```python
from build123d import *

# Parameters (mm, degrees)
F1_DEPTH = 12
F3_W     = 10
F3_H     = 2
F4_DEPTH = 43
F6_W     = 9
F6_H     = 4.75
F7_DEPTH = 69
F9_D     = 3.5
F9_DEPTH = 4
F9_TIP   = 1.0515060833


with BuildPart() as f1:
    # F0 (on Front) → F1 (new body)
    with BuildSketch(Plane.XZ):
        Polygon((29.6939597434, -5.2816280767), (-18.3060402566, -5.2816280767), (-18.3060402566, -14.0816280767), (29.6939597434, -14.0816280767), (29.6939597434, -10.5816280767), (27.6939597434, -10.5816280767), (27.6939597434, -11.5816280767), (-16.3060402566, -11.5816280767), (-16.3060402566, -8.2816280767), (27.6939597434, -8.2816280767), (27.6939597434, -9.2816280767), (29.6939597434, -9.2816280767), align=None)
    extrude(amount=F1_DEPTH)

    # F3 (on offset) → F4 (cut)
    with BuildSketch(Plane(origin=(27.6939597434, 0, 0), x_dir=(0, -1, 0), z_dir=(-1, 0, 0))):
        with Locations((6, -7.5316280767)):
            Rectangle(F3_W, F3_H)
    extrude(amount=F4_DEPTH, mode=Mode.SUBTRACT)

    # F6 (on offset) → F7 (cut)
    with BuildSketch(Plane.YZ.offset(54.6939597434)):
        with Locations((-6, -12.9234550223)):
            Rectangle(F6_W, F6_H)
    extrude(amount=-F7_DEPTH, mode=Mode.SUBTRACT)

    # F9
    with Locations(Plane(origin=(-18.3060402566, 0, 0), x_dir=(0, -1, 0), z_dir=(-1, 0, 0))):
        with Locations((6, -9.9316280767)):
            Hole(F9_D / 2, depth=F9_DEPTH)
            with Locations((0, 0, -(F9_DEPTH + F9_TIP / 2))):  # 118° drill point
                Cone(0, F9_D / 2, F9_TIP, mode=Mode.SUBTRACT)


solid = f1.part
```
Work out the finished part from the listing and answer in its coordinate system (mm). A direction names the side the tool comes from. Give positions to 0.01 mm unless a question says otherwise; leave off trailing zeros. Loops run counter-clockwise (first coordinate to the right, second up) from the corner with the lowest first, then second, coordinate; pieces in that order, holes last. Notation, with made-up numbers: M 47,-11 L 94,-11 A18 cw 94,-3 Z; hole C -16.75,-18 d3. An arc over 180 degrees is marked long. One line per item, written item: value. Start each with the question number.
1. Determine the mould class of faces 4 (the face through (29, -6, -9.282)), 5 (the face through (-14.306, -6, -13)), 6 (the face through (5, 0, -8)), 7 (the face through (27.694, -6, -8)) for opening direction Y: released by +Y, released by -Y, zero draft, split by the parting line, or undercut.
2. Find section A-A (x = -10). Give the vertices of the cut face in (y, z), and give its area (3 significant figures).
3. Find section C-C (z = -7.25). Give the vertices of the cut face in (x, y), and give its area (3 significant figures).
4. Find section D-D (z = -11). Give the vertices of the cut face in (x, y), and give its area (3 significant figures).
5. Find section B-B (y = -6). Give the vertices of the cut face in (x, z).
6. Which of the six approach directions +Z, -Z, +X, -X, +Y, -Y give full straight-line access (tool end or side, diameter ignored) to faces 1 (the face through (-17.167, -7.389, -10.996)), 2 (the face through (6, -11, -7)), 3 (the face through (27.694, -1, -11))?
7. Each of these flat-tipped pins is pushed along its axis until it touches: P1, Ø2.5, axis at y = -3, z = -9.5, coming from the +X side; P2, Ø1.3, axis at y = -5, z = -13.5, coming from the +X side; P3, Ø3, axis at x = 15.5, y = -4.5, coming from the -Z side; P4, Ø1, axis at y = -9, z = -10.5, coming from the +X side. Where does it stop, or does it pass through?
8. Find the intervals of material crossed by probe 1 along Z at (x, y) = (-15.9, -6); probe 2 along X at (y, z) = (-9, -6.75); probe 3 along Y at (x, z) = (17.5, -7.75), in increasing order.
Reported:
1. face 4: zero draft
1. face 5: undercut
1. face 6: released by +Y
1. face 7: undercut
2. outline: M -12,-14.08 L -10.5,-14.08 L -10.5,-11.58 L -12,-11.58 Z; M -12,-8.28 L -11,-8.28 L -11,-6.53 L -1,-6.53 L -1,-8.28 L 0,-8.28 L 0,-5.28 L -12,-5.28 Z; M -1.5,-14.08 L 0,-14.08 L 0,-11.58 L -1.5,-11.58 Z
2. area: 26.0 mm²
3. outline: M -18.31,-12 L 29.69,-12 L 29.69,0 L -18.31,0 Z; hole M -15.31,-11 L 27.69,-11 L 27.69,-1 L -15.31,-1 Z
3. area: 146 mm²
4. outline: M -18.31,-12 L -16.31,-12 L -16.31,-7.39 L -18.31,-7.39 Z; M -18.31,-4.61 L -16.31,-4.61 L -16.31,0 L -18.31,0 Z; M 27.69,-12 L 29.69,-12 L 29.69,-10.5 L 27.69,-10.5 Z; M 27.69,-1.5 L 29.69,-1.5 L 29.69,0 L 27.69,0 Z
4. area: 24.5 mm²
5. outline: M -18.31,-14.08 L -14.31,-14.08 L -14.31,-11.68 L -18.31,-11.68 Z; M -18.31,-8.18 L -15.31,-8.18 L -15.31,-6.53 L 27.69,-6.53 L 27.69,-9.28 L 29.69,-9.28 L 29.69,-5.28 L -18.31,-5.28 Z
6. face 1: -X
6. face 2: none
6. face 3: +Y, -Y
7. P1: stops at x = 29.69
7. P2: stops at x = -14.31
7. P3: stops at z = -6.53
7. P4: stops at x = -16.31
8. probe 1: z = -14.08 to -11.68, -8.18 to -5.28
8. probe 2: x = -18.31 to -15.31, 27.69 to 29.69
8. probe 3: y = -12 to -11, -1 to 0
